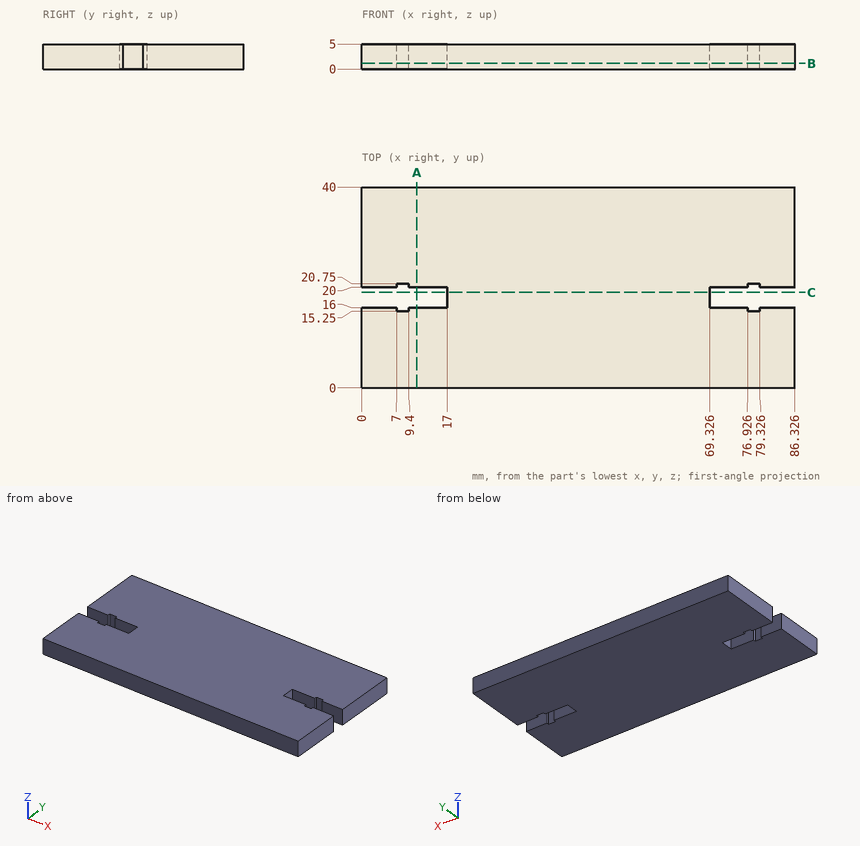
Study the drawing (mm; zero at the part's minimum x, y, z) and answer. Round coordinates to 2 decimals unless told otherwise and drop trailing zeros. Write each loop counter-clockwise with the first axis right and the second up, starting at its lowest first coordinate (ties: lowest second). Pieces come first, ordered by that corner, then holes. Notation, with made-up numbers: (17, 15) - (35, 15) arc R25 cw to (35, 48) - close; hole circle Ø6 at (49, 19.5). An arc over 180 degrees is marked (long way). Return JSON: item names as keys, results as strings. Group by question number.
Q1. The part is cut by section A-A on x = 11. Write down the section's boundary in (y, z).
Q2. This flat-tipped pin is pushed along its axis until it touches: pin 1 Ø2 at (y, z) = (18.5, 2) entering from +X. Where does it stop, or does it pass through?
Q3. The part is cut by section B-B on z = 1.15. Write down the section's boundary in (x, y).
Q4. Find the intervals of material crossed by L1, parallel to Y at x = 13, z = 4.65; L2, parallel to X at y = 18.5, z = 3.95, in increasing order.
Q5. The part is cut by section C-C on y = 19. Write down the section's boundary in (x, z).
Solved:
{
 "1": {"outline": "(0, 0) - (16, 0) - (16, 5) - (0, 5) - close; (20, 0) - (40, 0) - (40, 5) - (20, 5) - close"},
 "2": {"pin 1": "x = 69.33"},
 "3": {"outline": "(0, 0) - (86.33, 0) - (86.33, 16) - (79.33, 16) - (79.33, 15.25) - (76.93, 15.25) - (76.93, 16) - (69.33, 16) - (69.33, 20) - (76.93, 20) - (76.93, 20.75) - (79.33, 20.75) - (79.33, 20) - (86.33, 20) - (86.33, 40) - (0, 40) - (0, 20) - (7, 20) - (7, 20.75) - (9.4, 20.75) - (9.4, 20) - (17, 20) - (17, 16) - (9.4, 16) - (9.4, 15.25) - (7, 15.25) - (7, 16) - (0, 16) - close"},
 "4": {"L1": "0 to 16, 20 to 40", "L2": "17 to 69.33"},
 "5": {"outline": "(17, 0) - (69.33, 0) - (69.33, 5) - (17, 5) - close"}
}
